The listing builds one solid part. Answer for the finished solid, in the listing's coordinates (mm). Give positions to 0.01 mm unless a question says otherwise; leave off trailing zeros. Loops run counter-clockwise (first coordinate to the right, second up) from the corner with the lowest first, then second, coordinate; pieces in that order, holes last. Notation, with made-up numbers: M 66.25,76 L 121.25,76 A22 cw 121.25,91 Z; hole C -11.75,18 d3. An arc over 180 degrees is marked long. Return JSON: item names as keys, results as strings.
from build123d import *

# Parameters (mm, degrees)
SKETCH1_W           = 16.88
SKETCH1_H           = 12.7
BOSS_EXTRUDE1_DEPTH = 12.065
SKETCH3_R           = 3.25
BOSS_EXTRUDE2_DEPTH = 14.2
SKETCH4_R           = 1
CUT_EXTRUDE1_DEPTH  = 27.265


with BuildPart() as part:
    # Sketch1 → Boss-Extrude1 (new body)
    with BuildSketch(Plane(origin=(0, 0, 0), x_dir=(1, 0, 0), z_dir=(0, 1, 0))):
        with Locations((8.44, 6.35)):
            Rectangle(SKETCH1_W, SKETCH1_H)
    extrude(amount=BOSS_EXTRUDE1_DEPTH)

    # Sketch3 → Boss-Extrude2 (add)
    with BuildSketch(Plane(origin=(0, 12.065, 0), x_dir=(1, 0, 0), z_dir=(0, 1, 0))):
        with Locations((11.8, 6.35)):
            Circle(SKETCH3_R)
    extrude(amount=BOSS_EXTRUDE2_DEPTH)

    # Sketch4 → Cut-Extrude1 (cut, through all)
    with BuildSketch(Plane(origin=(0, 26.265, 0), x_dir=(1, 0, 0), z_dir=(0, 1, 0))):
        with Locations((11.8, 6.35)):
            Circle(SKETCH4_R)
    extrude(amount=-CUT_EXTRUDE1_DEPTH, mode=Mode.SUBTRACT)


solid = part.part
(1) The part is cut by section C-C (y = 23.75). Determine the outline of the cut face in (x, z).
Values follow:
{"outline": "C 11.8,-6.35 d6.5; hole C 11.8,-6.35 d2"}
(2) The part is cut by section D-D (z = -8.5). Determine the outline of the cut face in (x, y) (3 decimals).
Values follow:
{"outline": "M 0,0 L 16.88,0 L 16.88,12.065 L 14.237,12.065 L 14.237,26.265 L 9.363,26.265 L 9.363,12.065 L 0,12.065 Z"}
(3) The part is cut by section A-A (x = 11.8). Determine the outline of the cut face in (y, z) (3 decimals).
Values follow:
{"outline": "M 0,-12.7 L 12.065,-12.7 L 12.065,-9.6 L 26.265,-9.6 L 26.265,-7.35 L 0,-7.35 Z; M 0,-5.35 L 26.265,-5.35 L 26.265,-3.1 L 12.065,-3.1 L 12.065,0 L 0,0 Z"}
(4) Given pin 1 (6 mm diameter, centred on x = 13, y = 12, fed in from +Z); pin 2 (1.6 mm diameter, centred on x = 11.8, z = -6.35, fed in from +Y), each flat-ended and moving along its own axis, determine where each tip first touches the part or whether it passes through.
Values follow:
{"pin 1": "z = 0", "pin 2": "through"}
(5) The part is cut by section B-B (z = -6.35). Determine the outline of the cut face in (x, y) (3 decimals), and give its area (3 significant figures).
Values follow:
{"outline": "M 0,0 L 10.8,0 L 10.8,26.265 L 8.55,26.265 L 8.55,12.065 L 0,12.065 Z; M 12.8,0 L 16.88,0 L 16.88,12.065 L 15.05,12.065 L 15.05,26.265 L 12.8,26.265 Z", "area": "243 mm²"}
(6) Determine the mould class of faces 1 (the cylindrical face through (12.754, 13.316, -6.65)), 2 (the cylindrical face through (9.405, 19.066, -8.547)), 3 (the flat face through (8, 12.065, -6)) for opening direction X: released by +X, released by -X, zero draft, split by the parting line, or undercut.
Values follow:
{"face 1": "undercut", "face 2": "split by the parting line", "face 3": "zero draft"}
(7) Straight lines are drawn through the part: line 1 along X through (y, z) = (20.75, -6.35); line 2 along Z through (x, y) = (11.8, 13.25); line 3 along Y through (x, z) = (4.5, -10.75) (3 decimals). For each, find the intervals that lie inside material, in ascending order.
Values follow:
{"line 1": "8.55 to 10.8, 12.8 to 15.05", "line 2": "-9.6 to -7.35, -5.35 to -3.1", "line 3": "0 to 12.065"}
